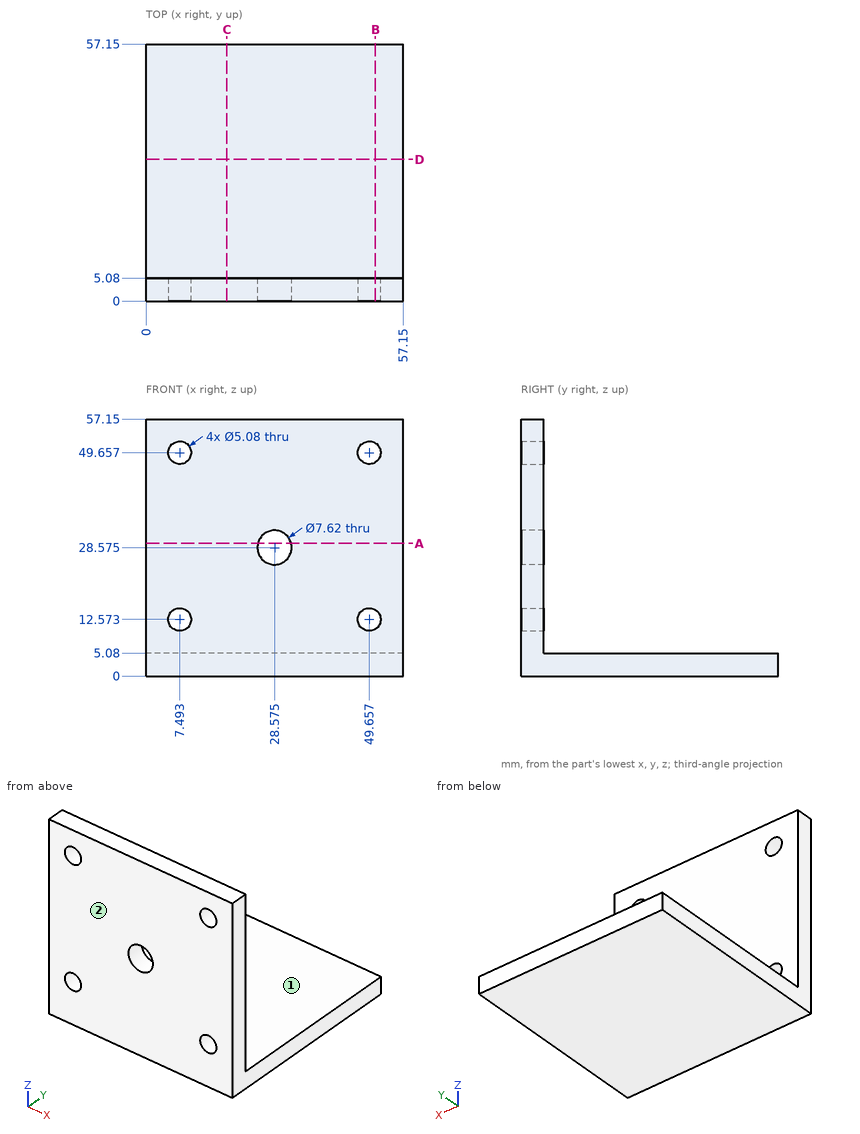
Here's the drawing with two shaded views (mm, measured from the low corner). I have some questions. A direction names the side the tool comes from. Coordinates: 2 decimals unless noted, no trailing zeros. Write each loop counter-clockwise with the first axis right and the second up, starting at its lowest first coordinate (ties: lowest second). Pieces come first, ordered by that corner, then holes. Notation, with made-up numbers: M -38,-23 L 3,-23 A19 cw 3,-18 Z; hole C 30.5,-19 d10. An arc over 180 degrees is marked long. Answer as CSV lines item,"result". Start each with the question number.
1) I want a section at A-A, the plane z = 29.5. Please give me the cut outline in (x, y).
2) For the marked faces 1 and 2, which set-ups out of +Z, -Z, +X, -X, +Y, -Y let a thin tool reach every point of the face, with its end or its side?
3) I want a section at C-C, the plane x = 18. Please give me the cut outline in (y, z).
4) Please list where these lines run through material, in increasing order: line 1 (Z direction, x = 25, y = 19.5); line 2 (Z direction, x = 50.5, y = 3). Write a range as from..to.
5) I want a section at B-B, the plane x = 51. Please give me the cut outline in (y, z), and give its area (3 significant figures).
6) I want a section at D-D, the plane y = 31.5. Please give me the cut outline in (x, z).
7) For P1, Ø9, axis at x = 28.575, z = 28.575, coming from the +Y side; P2, Ø3, axis at x = 42.5, y = 50, coming from the +Z side, each with a flat end and sliding along its axis, tell me the tip position at first contact or that it passes through.
Data:
1,outline,"M 0,0 L 24.88,0 L 24.88,5.08 L 0,5.08 Z; M 32.27,0 L 57.15,0 L 57.15,5.08 L 32.27,5.08 Z"
2,face 1,"+Z, +X, -X, +Y"
2,face 2,"+Z, -Z, +X, -X, -Y"
3,outline,"M 0,0 L 57.15,0 L 57.15,5.08 L 5.08,5.08 L 5.08,57.15 L 0,57.15 Z"
4,line 1,"z = 0..5.08"
4,line 2,"z = 0..10.18, 14.97..47.26, 52.05..57.15"
5,outline,"M 0,0 L 57.15,0 L 57.15,5.08 L 5.08,5.08 L 5.08,10.42 L 0,10.42 Z; M 0,14.73 L 5.08,14.73 L 5.08,47.5 L 0,47.5 Z; M 0,51.81 L 5.08,51.81 L 5.08,57.15 L 0,57.15 Z"
5,area,"511 mm^2"
6,outline,"M 0,0 L 57.15,0 L 57.15,5.08 L 0,5.08 Z"
7,P1,"stops at y = 5.08"
7,P2,"stops at z = 5.08"
